```python
from build123d import *

# Parameters (mm, degrees)
SKETCH1_W           = 70
SKETCH1_H           = 80
SKETCH1_R           = 1.75
BOSS_EXTRUDE1_DEPTH = 3
SKETCH2_R           = 1.75
CUT_EXTRUDE1_DEPTH  = 3


with BuildPart() as part:
    # Sketch1 → Boss-Extrude1 (new body)
    with BuildSketch(Plane(origin=(0, 0, 0), x_dir=(1, 0, 0), z_dir=(0, 1, 0))):
        with Locations((0, -6.5)):
            Rectangle(SKETCH1_W, SKETCH1_H)
        with Locations(Location((-20.5, 7.5, 0), (0, 0, 270))):
            Circle(SKETCH1_R, mode=Mode.SUBTRACT)
        with Locations(Location((-20.5, -7.5, 0), (0, 0, 90))):
            Circle(SKETCH1_R, mode=Mode.SUBTRACT)
        with Locations(Location((20.5, -7.5, 0), (0, 0, 270))):
            Circle(SKETCH1_R, mode=Mode.SUBTRACT)
        with Locations(Location((20.5, 7.5, 0), (0, 0, 90))):
            Circle(SKETCH1_R, mode=Mode.SUBTRACT)
    extrude(amount=BOSS_EXTRUDE1_DEPTH)

    # Sketch2 → Cut-Extrude1 (cut)
    with BuildSketch(Plane(origin=(0, 3, 0), x_dir=(1, 0, 0), z_dir=(0, 1, 0))):
        with Locations(Location((30, 28.5, 0), (0, 0, 270))):
            Circle(SKETCH2_R)
        with Locations(Location((-30, 28.5, 0), (0, 0, 90))):
            Circle(SKETCH2_R)
        with Locations(Location((30, -41.5, 0), (0, 0, 90))):
            Circle(SKETCH2_R)
        with Locations(Location((-30, -41.5, 0), (0, 0, 270))):
            Circle(SKETCH2_R)
    extrude(amount=-CUT_EXTRUDE1_DEPTH, mode=Mode.SUBTRACT)


solid = part.part
```
The model under review builds one solid part; all positions refer to its coordinate system, in mm. Give positions to 0.01 mm unless a question says otherwise; leave off trailing zeros. Loops run counter-clockwise (first coordinate to the right, second up) from the corner with the lowest first, then second, coordinate; pieces in that order, holes last. Notation, with made-up numbers: (33, 57) -> (50, 57) arc R21 cw to (50, 91) -> close; hole circle Ø5 at (46, 19). An arc over 180 degrees is marked (long way). Use CSV: the item, a comma, the result in double quotes.
1. Consider section A-A, the plane x = -30. Write out the cut boundary in (y, z).
Result:
outline,"(0, -33.5) -> (3, -33.5) -> (3, -30.25) -> (0, -30.25) -> close; (0, -26.75) -> (3, -26.75) -> (3, 39.75) -> (0, 39.75) -> close; (0, 43.25) -> (3, 43.25) -> (3, 46.5) -> (0, 46.5) -> close"
2. Consider section B-B, the plane z = -7.5. Write out the cut boundary in (x, y), then the cut area to 3 significant figures.
Result:
outline,"(-35, 0) -> (-22.25, 0) -> (-22.25, 3) -> (-35, 3) -> close; (-18.75, 0) -> (18.75, 0) -> (18.75, 3) -> (-18.75, 3) -> close; (22.25, 0) -> (35, 0) -> (35, 3) -> (22.25, 3) -> close"
area,"189 mm²"
3. To check wall thickness, follow probe 1 along X at (y, z) = (2.3, 7.5); probe 2 along X at (y, z) = (1.6, -28.5); probe 3 along Z at (x, y) = (-31.5, 1.95). State the ranges of each line that lie inside material, in increasing order. Write a range as from..to.
Result:
probe 1,"x = -35..-22.25, -18.75..18.75, 22.25..35"
probe 2,"x = -35..-31.75, -28.25..28.25, 31.75..35"
probe 3,"z = -33.5..-29.4, -27.6..40.6, 42.4..46.5"
4. The part is to be moulded in two halves that separate along Z. For faces 1 (the face through (35, 1, 7)), 2 (the face through (0, 1, 46.5)), 3 (the face through (18.765, 1.479, -7.272)), 4 (the face through (0, 1, -33.5)), say which applies: +Z half, -Z half, draft (parallel to the pull), parting line (faces both ways), or undercut.
Result:
face 1,"draft"
face 2,"+Z half"
face 3,"undercut"
face 4,"-Z half"
